Autodesk Inventor part; units mm, degrees
ref_plane "YZ Plane" through (0, 0, 0) normal (1, 0, 0) x (0, 1, 0)
ref_plane "XZ Plane" through (0, 0, 0) normal (0, 1, 0) x (-1, 0, 0)
ref_plane "XY Plane" through (0, 0, 0) normal (0, 0, 1) x (1, 0, 0)
sketch "スケッチ1" plane through (0, 0, 0) normal (1, 0, 0) x (0, 1, 0)
  circle A0 centre (0, 0) radius 3.5
  dimension "d0" = 7
extrude "押し出し1" add sketch "スケッチ1" along normal mid plane 18
sketch "スケッチ2" plane through (9, 0, 0) normal (1, 0, 0) x (0, 0, -1)
  circle A0 centre (0, 0) radius 1.75
  dimension "d3" = 3.5
extrude "押し出し2" cut sketch "スケッチ2" against normal through all
sketch "スケッチ3" plane through (9, 0, 0) normal (1, 0, 0) x (0, 0, -1)
  line L0 (-4.5, 4.5039) -> (-2.5, 4.5039)
  line L1 (-2.5, 4.5039) -> (-2.5, -4.5039)
  line L2 (-2.5, -4.5039) -> (-4.5, -4.5039)
  line L3 (-4.5, -4.5039) -> (-4.5, 4.5039)
  circle A0 centre (0, 0) radius 3.5
  line L4 (-4.5, 4.5039) -> (-2.5, -4.5039) construction
  line L5 (-2.5, 4.5039) -> (-4.5, -4.5039) construction
  point P0 (-3.5, 0)
extrude "押し出し3" cut sketch "スケッチ3" against normal through all contours L0 L1 A0 L2 L3 | L1 A0 picked at (-2.8262, -0.1289)
sketch "スケッチ5" plane through (9, -2.4495, 2.5) normal (0, 0, 1) x (1, 0, 0)
  circle A0 centre (-13, 2.6458) radius 1.5
  line L0 (-9, 2.4495) -> (-9, 9.8667) construction
  circle A1 centre (-5, 2.6458) radius 1.5
  dimension "d10" = 3
extrude "押し出し4" cut sketch "スケッチ5" against normal blind 3
thread "ねじ1"
thread "ねじ2"
properties part number "attachment2"
Geometry check sheet. Reference: the model listing, model coordinates, mm. A direction names the side the tool comes from. Coordinates: 2 decimals unless noted, no trailing zeros. Order: outer loops, then holes, each group sorted by start corner. A loop starts at its lowest first (then second) coordinate and runs counter-clockwise, first axis right, second up. Notation, with made-up numbers: M 46,71.25 L 53,71.25 A19 ccw 53,81.25 Z; hole C 10.25,55.25 d8. An arc over 180 degrees is marked long. Answer as a JSON object with one key per item and string values.
Q1. Cross-section at D-D on z = 0.75. Record the cut outline in (x, y).
Results are:
{"outline": "M -9,-3.42 L 9,-3.42 L 9,-1.58 L -9,-1.58 Z; M -9,1.58 L -4.58,1.58 A1.5 cw -3.42,1.58 L 3.42,1.58 A1.5 cw 4.58,1.58 L 9,1.58 L 9,3.42 L -9,3.42 Z"}
Q2. Scan lines: line 1 (X direction, y = 1.5, z = 1.5); line 2 (Y direction, x = -2, z = 0); line 3 (X direction, y = 1, z = 1.5). Record each from-to range of solid material in increasing order.
Results are:
{"line 1": "x = -9 to -4.74, -3.26 to 3.26, 4.74 to 9", "line 2": "y = -3.5 to -1.75, 1.75 to 3.5", "line 3": "x = -9 to -5.27, -2.73 to 2.73, 5.27 to 9"}
Q3. Cross-section at A-A on z = 0. Record the cut outline in (x, y).
Results are:
{"outline": "M -9,-3.5 L 9,-3.5 L 9,-1.75 L -9,-1.75 Z; M -9,1.75 L 9,1.75 L 9,3.5 L -9,3.5 Z"}
Q4. Tool access check on faces 1 (the cylindrical face through (4.81, 1.46, 1.94)), 2 (the flat face through (0, 0, 2.5)). Record the directions out of +Z, -Z, +X, -X, +Y, -Y that give a thin tool (end or side, any length) a straight path to the whole face; none if there is none.
Results are:
{"face 1": "+Z", "face 2": "+Z, +X, -X, +Y, -Y"}
Q5. Release check for a two-part mould opening along Z. For faces 3 (the cylindrical face through (-0.1, 0.1, -3.5)), 4 (the cylindrical face through (0.126, -0.67, -1.617)), 5 (the flat face through (-9, 0, -2)) record: released by +Z, released by -Z, zero draft, split by the parting line, or undercut.
Results are:
{"face 3": "split by the parting line", "face 4": "undercut", "face 5": "zero draft"}
Q6. Cross-section at B-B on y = -1. Record the cut outline in (x, z).
Results are:
{"outline": "M -9,-3.35 L 9,-3.35 L 9,-1.44 L -9,-1.44 Z; M -9,1.44 L -4.9,1.44 L -4.9,2.5 L -9,2.5 Z; M -3.1,1.44 L 3.1,1.44 L 3.1,2.5 L -3.1,2.5 Z; M 4.9,1.44 L 9,1.44 L 9,2.5 L 4.9,2.5 Z"}
